The model under review builds one solid part; all positions refer to its coordinate system, in mm. Give positions to 0.01 mm unless a question says otherwise; leave off trailing zeros. Loops run counter-clockwise (first coordinate to the right, second up) from the corner with the lowest first, then second, coordinate; pieces in that order, holes last. Notation, with made-up numbers: (85, -4) -> (116, -4) arc R9 cw to (116, 6) -> close; hole circle Ø1 at (55, 32). An arc over 180 degrees is marked (long way). Write each question's results on one line, items separated by ' | '. Start each with the question number.
Q1. We need section A-A (y = -3). Write out the cut boundary in (x, z), plus the area to 3 significant figures.
Q2. Insertion check: pin 1 Ø12 at (x, y) = (-21, -2.5) entering from +Z; pin 2 Ø5 at (x, y) = (9, -8.5) entering from +Z. Each pin has a flat end and moves straight along its axis. Give the tip position at first contact, or say it passes through.
Q3. Wall thickness on L1, parallel to Z at x = 12, y = -11.25; L2, parallel to X at y = -8.5, z = 23.5; L3, parallel to Z at x = -17, y = -22: over which ranges is each line inside the solid? List them lowest first. Write a range as [from, to].
Q4. We need section B-B (y = -23.5). Write out the cut boundary in (x, z), plus the area to 3 significant figures.
from build123d import *

# Parameters (mm, degrees)
F0_W     = 45.0788065791
F0_H     = 49.5671723038
F1_DEPTH = 25.4
F3_R     = 5.08


# Not quite as in the source:
# - a feature of the source that left no trace in its solid (it failed there, or was rolled back) is left out


with BuildPart() as f1:
    # F0 (on Front) → F1 (new body)
    with BuildSketch(Plane.XZ):
        with Locations((-4.0004998446, -2.9271943495)):
            Rectangle(F0_W, F0_H)
        Polygon((-5.2689509466, 43.1273430586), (-26.5399031341, 21.8563918024), (18.538903445, 21.8563918024), align=None)
    extrude(amount=F1_DEPTH)

    # F3
    f3_edges = [f1.edges().sort_by_distance(p)[0] for p in [
        (-15.904427, -25.4, 32.491867),
        (-26.539903, -25.4, -2.927194),
        (-4.0005, -25.4, -27.710781),
        (18.538903, -25.4, -2.927194),
        (6.634976, -25.4, 32.491867),
        (18.538903, -12.7, 21.856392),
        (-5.268951, -12.7, 43.127343),
    ]]
    fillet(f3_edges, radius=F3_R)


solid = f1.part
Output:
1) outline: (-26.54, -27.71) -> (18.54, -27.71) -> (18.54, 19.58) arc R5.08 ccw to (16.84, 23.37) -> (-1.69, 39.93) arc R5.08 ccw to (-8.66, 39.73) -> (-26.54, 21.86) -> close | area: 2,710 mm2
2) pin 1: z = 33.4 | pin 2: z = 32.61
3) L1: [-27.71, 27.7] | L2: [-24.9, 16.7] | L3: [-27.42, 30.99]
4) outline: (-25.42, -26.59) -> (17.42, -26.59) -> (17.42, 19.58) arc R3.96 ccw to (16.1, 22.54) -> (-2.43, 39.09) arc R3.96 ccw to (-7.87, 38.94) -> (-25.42, 21.39) -> close | area: 2,480 mm2
